Could you check a few things on this model? Use its own coordinates, in mm. Round coordinates to 2 decimals unless told otherwise and drop trailing zeros. Loops run counter-clockwise (first coordinate to the right, second up) from the corner with the lowest first, then second, coordinate; pieces in that order, holes last. Notation, with made-up numbers: M 39.5,-13 L 92.5,-13 A7 cw 92.5,0 Z; hole C 74,-40 d3. An arc over 180 degrees is marked long. One line per item, written item: value. Start each with the question number.
Q1. Imagine slicing it at A-A (z = 0). Please give me the cut outline in (x, y) (3 decimals), then the cut area to 3 significant figures.
Q2. Imagine slicing it at C-C (y = 1.25). Please give me the cut outline in (x, z) (3 decimals).
Q3. I'm going to push flat-ended pins straight in: pin 1 Ø1.5 at (x, y) = (-11.5, 1) entering from -Z; pin 2 Ø1 at (x, y) = (49, 2) entering from +Z; pin 3 Ø1 at (x, y) = (-62.5, 2) entering from -Z; pin 4 Ø5 at (x, z) = (0, -8) entering from -Y. Where does each tip first touch, or does it pass through?
Q4. Imagine slicing it at B-B (x = 51). Give the number of separate pieces and of enclosed holes in the cut face, then the cut area to 3 significant figures.
Q5. Imagine slicing it at D-D (z = 28). Please give me the cut outline in (x, y) (3 decimals), then the cut area to 3 significant figures.
Q6. Please list where these lines run through material, in increasing order: line 1 along Z through (x, y) = (79, 2.9); line 2 along X through (y, z) = (2.4, 9); line 3 along Z through (x, y) = (-34, 1.6).
from build123d import *

# Parameters (mm, degrees)
SKETCH4_R           = 128.5748
BOSS_EXTRUDE1_DEPTH = 3.175
CUT_EXTRUDE2_DEPTH  = 182.859943404
SCREW_HOLES_R       = 1.513296856
SCREW_HOLES_R_2     = 5.08
MIDDLE_HOLES_DEPTH  = 182.859943404
FILLETMIDDLE_R      = 20.32
FILLETSIDES_R       = 5.08


with BuildPart() as part:
    # Sketch4 → Boss-Extrude1 (new body)
    with BuildSketch(Plane(origin=(0, 0, 0), x_dir=(1, 0, 0), z_dir=(0, 1, 0))):
        with Locations(Location((0, 0, 0), (0, 0, 270))):
            Circle(SKETCH4_R)
    extrude(amount=BOSS_EXTRUDE1_DEPTH)

    # Sketch1 → Cut-Extrude2 (cut, through all)
    with BuildSketch(Plane(origin=(0, 0, 0), x_dir=(1, 0, 0), z_dir=(0, 1, 0))):
        with BuildLine():
            Line((-14.549677831, 6.35), (-125.238921027, 6.35))
            ThreePointArc((-125.238921027, 6.35), (0, 125.3998), (125.238921027, 6.35))
            Line((125.238921027, 6.35), (14.549677831, 6.35))
            ThreePointArc((14.549677831, 6.35), (0, 15.875), (-14.549677831, 6.35))
        make_face()
        with BuildLine():
            Line((125.238921027, -6.35), (14.549677831, -6.35))
            ThreePointArc((14.549677831, -6.35), (11.225320151, -11.225320151), (6.35, -14.549677831))
            Line((6.35, -14.549677831), (6.35, -125.238921027))
            ThreePointArc((6.35, -125.238921027), (88.671048939, -88.671048939), (125.238921027, -6.35))
        make_face()
        with BuildLine():
            Line((-6.35, -14.549677831), (-6.35, -125.238921027))
            ThreePointArc((-6.35, -125.238921027), (-88.671048939, -88.671048939), (-125.238921027, -6.35))
            Line((-125.238921027, -6.35), (-14.549677831, -6.35))
            ThreePointArc((-14.549677831, -6.35), (-11.225320151, -11.225320151), (-6.35, -14.549677831))
        make_face()
    extrude(amount=CUT_EXTRUDE2_DEPTH, mode=Mode.SUBTRACT)

    # Screw holes → middle holes (cut, through all)
    with BuildSketch(Plane(origin=(0, 0, 0), x_dir=(1, 0, 0), z_dir=(0, 1, 0))):
        with Locations(Location((0, 8, 0), (0, 0, 270))):
            Circle(SCREW_HOLES_R)
        with Locations(Location((0, -8, 0), (0, 0, 270))):
            Circle(SCREW_HOLES_R)
        with Locations(Location((0, 0, 0), (0, 0, 270))):
            Circle(SCREW_HOLES_R_2)
    extrude(amount=MIDDLE_HOLES_DEPTH, mode=Mode.SUBTRACT)

    # Filletmiddle
    # the kernel refuses this fillet: 20.32 mm, written as the material it adds along each edge
    with BuildSketch(Plane(origin=(-14.549677831, 0, -6.35), x_dir=(-1, 0, 0), z_dir=(0, 1, 0)), Plane(origin=(14.549677831, 0, 6.35), x_dir=(1, 0, 0), z_dir=(0, 1, 0)), Plane(origin=(-6.35, 0, 14.549677831), x_dir=(0, 0, 1), z_dir=(0, 1, 0))) as filletmiddle_piece_1:
        with BuildLine():
            CenterArc((9.920490231, -20.32), FILLETMIDDLE_R, 90, 42.536898363)
            ThreePointArc((-3.81714798, -5.347368421), (-1.628915718, -2.873314556), (0, 0))
            Line((0, 0), (9.920490231, 0))
        make_face()
    extrude(amount=3.175)
    with BuildSketch(Plane(origin=(14.549677831, 0, -6.35), x_dir=(1, 0, 0), z_dir=(0, 1, 0)), Plane(origin=(-14.549677831, 0, 6.35), x_dir=(-1, 0, 0), z_dir=(0, 1, 0))) as filletmiddle_piece_2:
        with BuildLine():
            CenterArc((9.920490231, 20.32), FILLETMIDDLE_R, 227.463101637, 42.536898363)
            ThreePointArc((-3.81714798, 5.347368421), (-1.628915718, 2.873314556), (0, 0))
            Line((0, 0), (9.920490231, 0))
        make_face()
    extrude(amount=3.175)
    with BuildSketch(Plane(origin=(6.35, 0, 14.549677831), x_dir=(0.8139062748674819, 0, -0.580996192527403), z_dir=(0, 1, 0))) as filletmiddle_piece_3:
        with BuildLine():
            CenterArc((10.774808453, -19.880191881), FILLETMIDDLE_R, 101.942461579, 42.536898363)
            Line((-5.763767052, -8.074349249), (0, 0))
            ThreePointArc((0, 0), (3.285002577, -0.343600093), (6.570005154, 0))
        make_face()
    extrude(amount=3.175)

    # Filletsides
    filletsides_edges = [part.edges().sort_by_distance(p)[0] for p in [
        (125.238921027, 1.5875, -6.35),
        (-125.238921027, 1.5875, -6.35),
        (6.35, 1.5875, 125.238921027),
        (125.238921027, 1.5875, 6.35),
        (-125.238921027, 1.5875, 6.35),
        (-6.35, 1.5875, 125.238921027),
    ]]
    fillet(filletsides_edges, radius=FILLETSIDES_R)


solid = part.part
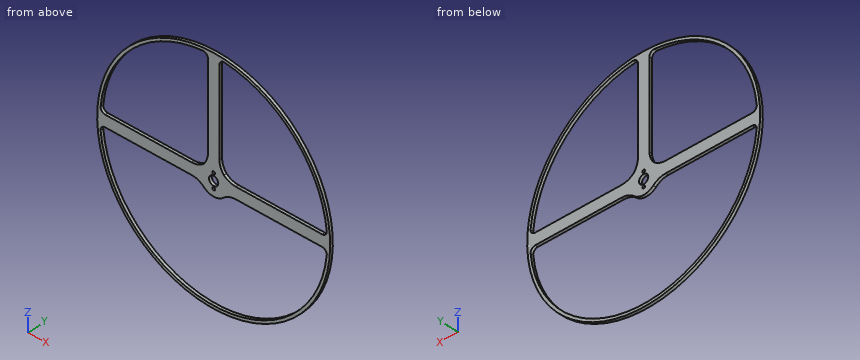
Report:
1. outline: M -128.575,0 L -5.08,0 L -5.08,3.175 L -128.575,3.175 Z; M 5.08,0 L 128.575,0 L 128.575,3.175 L 5.08,3.175 Z
1. area: 784 mm²
2. outline: C 0,0 d257.15; hole M -124.833,-11.913 A125.4 ccw 124.833,-11.913 A5.08 ccw 119.776,-6.35 L 24.47,-6.35 A20.32 ccw 10.733,-11.697 A15.875 cw -10.733,-11.697 A20.32 ccw -24.47,-6.35 L -119.776,-6.35 A5.08 ccw Z; hole M -124.833,11.913 A5.08 ccw -119.776,6.35 L -24.47,6.35 A20.32 ccw -11.244,11.244 A20.32 ccw -6.35,24.47 L -6.35,119.776 A5.08 ccw -11.913,124.833 A125.4 ccw Z; hole C 0,0 d10.16; hole C 0,-8 d3.027; hole C 0,8 d3.027; hole M 6.35,24.47 A20.32 ccw 11.244,11.244 A20.32 ccw 24.47,6.35 L 119.776,6.35 A5.08 ccw 124.833,11.913 A125.4 ccw 11.913,124.833 A5.08 ccw 6.35,119.776 Z
3. pin 1: stops at z = -128.12
3. pin 2: stops at z = 119.08
3. pin 3: stops at z = -112.64
3. pin 4: stops at y = 0
4. separate pieces: 3
4. enclosed holes: 0
4. area: 62.3 mm²
5. outline: M -125.489,0 L -122.234,0 L -122.234,3.175 L -125.489,3.175 Z; M -6.35,0 L 6.35,0 L 6.35,3.175 L -6.35,3.175 Z; M 122.234,0 L 125.489,0 L 125.489,3.175 L 122.234,3.175 Z
5. area: 61.0 mm²
6. line 1: z = -101.44 to -97.39, -6.35 to 6.35, 97.39 to 101.44
6. line 2: x = -128.26 to -124.24, -14.44 to -1.14, 1.14 to 14.44, 124.24 to 128.26
6. line 3: z = -124 to -120.7, -6.35 to 6.35, 120.7 to 124
